Read the model definition and answer for the solid it produces. Units are mm, in the model's axes. A direction names the side the tool comes from. Coordinates: 2 decimals unless noted, no trailing zeros. Loops run counter-clockwise (first coordinate to the right, second up) from the corner with the lowest first, then second, coordinate; pieces in that order, holes last. Notation, with made-up numbers: (4, -17.5) -> (22, -17.5) arc R16 cw to (22, -10.5) -> close; hole circle Ø6 at (-30.5, -36). An arc over 180 degrees is marked (long way). Answer in a Markdown table with one row per item.
```python
from build123d import *

# Parameters (mm, degrees)
SKETCH1_W           = 45
SKETCH1_H           = 25.4
BOSS_EXTRUDE1_DEPTH = 7.2
FILLET1_R           = 9
SKETCH5_R           = 2.25
SKETCH5_R_2         = 0.8
CUT_EXTRUDE1_DEPTH  = 32.680717235
CUT_EXTRUDE2_DEPTH  = 4
SKETCH7_R           = 43
BOSS_EXTRUDE2_DEPTH = 7
CUT_EXTRUDE5_REACH  = 89.211
SKETCH10_R          = 4.070055362
CUT_EXTRUDE6_REACH  = 85.227
SKETCH11_R          = 2.2
SKETCH11_W          = 41
SKETCH11_H          = 21


with BuildPart() as part:
    # Sketch1 → Boss-Extrude1 (new body)
    with BuildSketch(Plane(origin=(0, 0, 0), x_dir=(1, 0, 0), z_dir=(0, 1, 0))):
        with Locations((-5.305107108, -0.668016429)):
            Rectangle(SKETCH1_W, SKETCH1_H)
    extrude(amount=BOSS_EXTRUDE1_DEPTH)

    # Fillet1
    fillet1_edges = [part.edges().sort_by_distance(p)[0] for p in [
        (-27.805107108, 3.6, -12.031983571),
        (-27.805107108, 3.6, 13.368016429),
    ]]
    fillet(fillet1_edges, radius=FILLET1_R)

    # Sketch5 → Cut-Extrude1 (cut, through all)
    with BuildSketch(Plane(origin=(0, 7.2, 0), x_dir=(1, 0, 0), z_dir=(0, 1, 0))):
        with Locations(Location((-15.105107108, -0.668016429, 0), (0, 0, 270))):
            Circle(SKETCH5_R)
        with Locations(Location((-19.105107108, -0.668016429, 0), (0, 0, 270))):
            Circle(SKETCH5_R_2)
        with Locations(Location((-11.105107108, -0.668016429, 0), (0, 0, 270))):
            Circle(SKETCH5_R_2)
    extrude(amount=-CUT_EXTRUDE1_DEPTH, mode=Mode.SUBTRACT)

    # Sketch6 → Cut-Extrude2 (cut)
    with BuildSketch(Plane.XZ):
        with BuildLine():
            Line((-19.105107108, 3.818299004), (-11.105107108, 3.818299004))
            ThreePointArc((-11.105107108, 3.818299004), (-7.954824533, 0.668016429), (-11.105107108, -2.482266146))
            Line((-11.105107108, -2.482266146), (-19.105107108, -2.482266146))
            ThreePointArc((-19.105107108, -2.482266146), (-22.255389683, 0.668016429), (-19.105107108, 3.818299004))
        make_face()
    extrude(amount=-CUT_EXTRUDE2_DEPTH, mode=Mode.SUBTRACT)

    # Sketch7 → Boss-Extrude2 (add)
    with BuildSketch(Plane(origin=(17.194892892, 0, 0), x_dir=(0, 0, -1), z_dir=(1, 0, 0))):
        with Locations((0, -12.251447975)):
            Circle(SKETCH7_R)
    extrude(amount=BOSS_EXTRUDE2_DEPTH)

    # Sketch10 → Cut-Extrude5 (cut, up to next)
    with BuildSketch(Plane(origin=(24.194892892, 0, 0), x_dir=(0, 0, -1), z_dir=(1, 0, 0)), mode=Mode.PRIVATE) as cut_extrude5_sk1:
        with Locations((0, -12.251447975)):
            Circle(SKETCH10_R)
    cut_extrude5_tool1 = extrude(cut_extrude5_sk1.sketch, amount=-CUT_EXTRUDE5_REACH, mode=Mode.PRIVATE) & part.part
    add(cut_extrude5_tool1.solids().sort_by_distance((24.194893, -12.251448, 0))[0], mode=Mode.SUBTRACT)

    # Sketch11 → Cut-Extrude6 (cut, up to next)
    with BuildSketch(Plane.ZY.offset(-17.194892892), mode=Mode.PRIVATE) as cut_extrude6_sk1:
        with Locations((35.189613301, -7.251447975)):
            Circle(SKETCH11_R)
    cut_extrude6_tool1 = extrude(cut_extrude6_sk1.sketch, amount=-CUT_EXTRUDE6_REACH, mode=Mode.PRIVATE) & part.part
    # Sketch11 → Cut-Extrude6 (cut, up to next)
    with BuildSketch(Plane.ZY.offset(-17.194892892), mode=Mode.PRIVATE) as cut_extrude6_sk2:
        with Locations((35.189613301, -17.251447975)):
            Circle(SKETCH11_R)
    cut_extrude6_tool2 = extrude(cut_extrude6_sk2.sketch, amount=-CUT_EXTRUDE6_REACH, mode=Mode.PRIVATE) & part.part
    # Sketch11 → Cut-Extrude6 (cut, up to next)
    with BuildSketch(Plane.ZY.offset(-17.194892892), mode=Mode.PRIVATE) as cut_extrude6_sk3:
        with Locations((-14.589613301, -7.251447975)):
            Circle(SKETCH11_R)
    cut_extrude6_tool3 = extrude(cut_extrude6_sk3.sketch, amount=-CUT_EXTRUDE6_REACH, mode=Mode.PRIVATE) & part.part
    # Sketch11 → Cut-Extrude6 (cut, up to next)
    with BuildSketch(Plane.ZY.offset(-17.194892892), mode=Mode.PRIVATE) as cut_extrude6_sk4:
        with Locations((-14.589613301, -17.251447975)):
            Circle(SKETCH11_R)
    cut_extrude6_tool4 = extrude(cut_extrude6_sk4.sketch, amount=-CUT_EXTRUDE6_REACH, mode=Mode.PRIVATE) & part.part
    # Sketch11 → Cut-Extrude6 (cut, up to next)
    with BuildSketch(Plane.ZY.offset(-17.194892892), mode=Mode.PRIVATE) as cut_extrude6_sk5:
        with Locations((10.3, -12.251447975)):
            Rectangle(SKETCH11_W, SKETCH11_H)
    cut_extrude6_tool5 = extrude(cut_extrude6_sk5.sketch, amount=-CUT_EXTRUDE6_REACH, mode=Mode.PRIVATE) & part.part
    add(cut_extrude6_tool1.solids().sort_by_distance((17.194893, -7.251448, 35.189613))[0], mode=Mode.SUBTRACT)
    add(cut_extrude6_tool2.solids().sort_by_distance((17.194893, -17.251448, 35.189613))[0], mode=Mode.SUBTRACT)
    add(cut_extrude6_tool3.solids().sort_by_distance((17.194893, -7.251448, -14.589613))[0], mode=Mode.SUBTRACT)
    add(cut_extrude6_tool4.solids().sort_by_distance((17.194893, -17.251448, -14.589613))[0], mode=Mode.SUBTRACT)
    add(cut_extrude6_tool5.solids().sort_by_distance((17.194893, -12.251448, 10.3))[0], mode=Mode.SUBTRACT)


solid = part.part
```
1. A cutting plane is placed at A-A on z = -5.5. Give the vertices of the cut face in (x, y).
A:
| item | result |
|---|---|
| outline | (-27.46, 0) -> (17.19, 0) -> (17.19, -1.75) -> (24.19, -1.75) -> (24.19, 30.4) -> (17.19, 30.4) -> (17.19, 7.2) -> (-27.46, 7.2) -> close; (17.19, -54.9) -> (24.19, -54.9) -> (24.19, -22.75) -> (17.19, -22.75) -> close |
2. A cutting plane is placed at C-C on z = 12. Give the vertices of the cut face in (x, y).
A:
| item | result |
|---|---|
| outline | (-23.58, 0) -> (17.19, 0) -> (17.19, -1.75) -> (24.19, -1.75) -> (24.19, 29.04) -> (17.19, 29.04) -> (17.19, 7.2) -> (-23.58, 7.2) -> close; (17.19, -53.54) -> (24.19, -53.54) -> (24.19, -22.75) -> (17.19, -22.75) -> close |
3. The mould has two halves that part along Z. Classify faces 1 (the cylindrical face through (-22.255, 1.972, 0.599)), 2 (the flat face through (-1, 4, 13.368)), 3 (the flat face through (-6, 7.2, 0)), 4 (the cylindrical face through (20.65, -38.42, 34.12)): pulls with the +Z half, pulls with the -Z half, needs draft (parallel to the pull), parting line crosses it, or undercut.
A:
| item | result |
|---|---|
| face 1 | undercut |
| face 2 | pulls with the +Z half |
| face 3 | needs draft |
| face 4 | parting line crosses it |
4. A tool of negligible diameter and unlimited length cuts with its end or side. For faces 5 (the flat face through (-15, 2, 3.818)), 6 (the flat face through (-1, 4, -12.032)), 7 (the flat face through (-6, 0, 0)), from which of +Z, -Z, +X, -X, +Y, -Y can it reach the whole face along a straight path? Write none if from no direction.
A:
| item | result |
|---|---|
| face 5 | -Y |
| face 6 | -Z, -X, +Y, -Y |
| face 7 | +Z, -Z, -X, -Y |
5. Find the intervals of material crossed by probe 1 along X at (y, z) = (3, -3.5); probe 2 along Y at (x, z) = (7, -3.5); probe 3 along X at (y, z) = (-45, 3), in increasing order.
A:
| item | result |
|---|---|
| probe 1 | x = -27.79 to 24.19 |
| probe 2 | y = 0 to 7.2 |
| probe 3 | x = 17.19 to 24.19 |
6. A cutting plane is placed at B-B on x = -5. Give the vertices of the cut face in (y, z), and give its area (3 significant figures).
A:
| item | result |
|---|---|
| outline | (0, -12.03) -> (7.2, -12.03) -> (7.2, 13.37) -> (0, 13.37) -> close |
| area | 183 mm2 |
7. A cutting plane is placed at D-D on y = 19. Give the vertices of the cut face in (x, z), and give its area (3 significant figures).
A:
| item | result |
|---|---|
| outline | (17.19, -29.54) -> (24.19, -29.54) -> (24.19, 29.54) -> (17.19, 29.54) -> close |
| area | 413 mm2 |
8. Given pin 1 Ø5 at (y, z) = (-17.25, 35.19) entering from -X; pin 2 Ø5 at (x, z) = (-15.11, 0.67) entering from +Y; pin 3 Ø1.5 at (x, z) = (-3.5, 5.5) entering from -Y; pin 4 Ø3 at (y, z) = (-20, 30) entering from +X, each flat-ended and moving along its own axis, determine where each tip first touches the part or whether it passes through.
A:
| item | result |
|---|---|
| pin 1 | stops at x = 17.19 |
| pin 2 | stops at y = 7.2 |
| pin 3 | stops at y = 0 |
| pin 4 | stops at x = 24.19 |
